Autodesk Inventor part; units mm, degrees
ref_plane "YZ Plane" through (0, 0, 0) normal (1, 0, 0) x (0, 1, 0)
ref_plane "XZ Plane" through (0, 0, 0) normal (0, 1, 0) x (-1, 0, 0)
ref_plane "XY Plane" through (0, 0, 0) normal (0, 0, 1) x (1, 0, 0)
sketch "Boceto1" plane through (0, 0, 0) normal (0, 0, 1) x (1, 0, 0)
  line L0 (30, -83.65) -> (30, 0)
  line L1 (0, 0) -> (30, 0)
  line L2 (0, 0) -> (0, -83.65)
  line L3 (0, -83.65) -> (30, -83.65)
  line L4 (-13.92, -24.65) -> (-9.92, -24.65)
  line L5 (30, -83.65) -> (-55, -83.65)
  line L6 (-55, -83.65) -> (-55, -24.65)
  line L7 (-55, -24.65) -> (30, -24.65)
  line L8 (30, -24.65) -> (30, -83.65)
  line L9 (-55, -24.65) -> (-55, -21.65)
  line L10 (-55, -21.65) -> (30, -21.65)
  line L11 (0, -83.65) -> (10, -83.65)
  line L12 (10, -83.65) -> (10, -21.65)
  circle A0 centre (5, -78.65) radius 2.1
  circle A1 centre (5, -26.65) radius 2.1
  dimension "d0" = 85
  dimension "d1" = 59
  dimension "d2" = 3
  dimension "d5" = 10
extrude "Extrusión1" add sketch "Boceto1" along normal blind 6 contours L3 L2 L7 A1 L12 | L7 A1 L2 L10 L12 | L5 L6 L7 L4 L2 | A1 L7 | L7 A1 | L7 L4 L9 L10 L2 | A0
sketch "Boceto2" plane through (0, 0, 6) normal (0, 0, 1) x (1, 0, 0)
  line L0 (10, -83.65) -> (10, -21.65)
  line L1 (-55, -83.65) -> (10, -83.65)
  line L2 (10, -21.65) -> (-55, -21.65)
  point P0 (0, 0)
  point P1 (5, -78.65)
  point P2 (5, -26.65)
  dimension "d6" = 5
  dimension "d7" = 5
  dimension "d8" = 5
  dimension "d9" = 5
hole "Agujero1" at (5, -78.65, 6) at (5, -26.65, 6) direction (0, 0, -1) diameter 3.2 end through all
sketch "Boceto3" plane through (0, 0, 0) normal (0, 0, -1) x (-1, 0, 0)
  circle A0 centre (-5, -78.65) radius 2.1
  circle A1 centre (-5, -26.65) radius 2.1
  line L0 (-12, 0) -> (-12, -7.15)
  line L1 (-12, -7.15) -> (-30, -7.15)
  line L2 (-30, -7.15) -> (-30, -83.65)
  line L3 (0, -83.65) -> (-30, -83.65)
  line L4 (0, -83.65) -> (0, 0)
  line L5 (0, 0) -> (-12, 0)
  line L6 (20.12, -21.65) -> (-10, -21.65)
  line L7 (-10, -21.65) -> (-10, -83.65)
  circle A2 centre (-5, -26.65) radius 1.6
  circle A3 centre (-5, -78.65) radius 1.6
  circle A4 centre (-5, -26.65) radius 1.6
  circle A5 centre (-5, -78.65) radius 1.6
  line L8 (55, -21.65) -> (55, -83.65)
  line L9 (-10, -21.65) -> (55, -21.65)
  line L10 (-10, -83.65) -> (-10, -21.65)
  line L11 (55, -83.65) -> (-10, -83.65)
  line L12 (-10, -83.65) -> (20.12, -83.65)
  line L13 (20.12, -83.65) -> (20.12, -21.65)
  point P0 (0, -21.65)
extrude "Extrusión2" cut sketch "Boceto3" against normal blind 3 contours A0 | A1 | L5 L4 L6 L7 L3 L2 L1 L0 | L6 L13 L11 L4 | L4 L3 L7 L6 | L9 L8 L11 L13 | A2 | A3
sketch "Boceto4" plane through (-55, -21.65, 6) normal (0, 1, 0) x (1, 0, 0)
  line L0 (65, 3) -> (0, 3)
  line L1 (0, 3) -> (0, 0)
  line L2 (65, 0) -> (0, 0)
  line L3 (65, 3) -> (65, 0)
  line L4 (0, 0) -> (65, 0)
  line L5 (65, 0) -> (65, 6)
  line L6 (65, 6) -> (0, 6)
  line L7 (0, 6) -> (0, 0)
  point P0 (55, 6)
extrude "Extrusión3" add sketch "Boceto4" along normal blind 5
sketch "Boceto5" plane through (-55, -83.65, 3) normal (-1, 0, 0) x (0, 0, 1)
  line L0 (-69, 62) -> (-69, 59)
  line L1 (-3, 59) -> (-69, 59)
  line L2 (-3, 59) -> (-3, 62)
  line L3 (-3, 62) -> (-69, 62)
  line L4 (0, 62) -> (0, 0)
  line L5 (0, 0) -> (3, 0)
  line L6 (3, 0) -> (3, 67)
  line L7 (-3, 67) -> (3, 67)
  line L8 (-3, 62) -> (-3, 67)
  line L9 (-3, 62) -> (0, 62)
  line L10 (-3, 59) -> (3, 59)
  line L11 (3, 59) -> (3, 62)
  line L12 (3, 62) -> (-3, 62)
  line L13 (-3, 62) -> (-3, 59)
  point P0 (-3, 83.65)
  point P1 (0, 59)
extrude "Extrusión4" cut sketch "Boceto5" against normal blind 33.88 contours L12 L6 L10 L4
sketch "Boceto6" plane through (-55, -16.65, 6) normal (0, 1, 0) x (1, 0, 0)
  line L0 (0, 6) -> (0, 0)
  line L1 (0, 0) -> (65, 0)
  line L2 (65, 0) -> (65, 6)
  line L3 (65, 6) -> (0, 6)
  line L4 (0, 0) -> (0, 3)
  line L5 (0, 3) -> (3, 3)
  circle A0 centre (3, 3) radius 2.1
  line L6 (33.88, 3) -> (33.88, 0)
  line L7 (33.88, 3) -> (30.88, 3)
  circle A1 centre (30.88, 3) radius 2.1
  dimension "d34" = 3
  dimension "d35" = 4.2
  dimension "d36" = 4.2
hole "Agujero2" at (-52, -16.65, 3) at (-24.12, -16.65, 3) direction (0, -1, 0) diameter 4.2 depth 5
properties part number "Lateral izquierdo"
Input: part model. Units: mm. Frame: model coordinates. A direction names the side the tool comes from. Coordinates: 2 decimals unless noted, no trailing zeros. Write each loop counter-clockwise with the first axis right and the second up, starting at its lowest first coordinate (ties: lowest second). Pieces come first, ordered by that corner, then holes. Notation, with made-up numbers: M 84,-6 L 135,-6 A15 ccw 135,16 Z; hole C 79,28 d10. An arc over 180 degrees is marked long. Answer as a JSON object with one key per item and string values. Group by question number.
(1) Section A-A on x = 5. Output: boundary loops of the cut face in (y, z), plus the area to 3 significant figures.
(2) Section C-C on x = -40. Output: boundary loops of the cut face in (y, z).
(3) Mould query, pull axis Y, two halves, no side actions, for faces 4 (the face through (4.93, -77.05, 4.48)), 5 (the face through (-22.257, -19.185, 3.969)), 6 (the face through (-23, -16.65, 1)). Classes: pulls with the +Y half, pulls with the -Y half, needs draft (parallel to the pull), parting line crosses it, or undercut.
(4) Ray query, line 1 along X through (y, z) = (-18.1, 3); line 2 along Y through (x, z) = (5, 3.75); line 3 along X through (y, z) = (-26.65, 4). Return the intervals inside material, ascending. Write a range as [from, to].
(5) Section B-B on y = -26.65. Output: boundary loops of the cut face in (x, z).
(6) Section D-D on x = -24.12. Output: boundary loops of the cut face in (y, z).
(7) Set-up query: faces 1 (the face through (-22, -52, 3)), 2 (the face through (-23, -21.65, 1)), 3 (the face through (-21.12, -23, 4)). Return all of +Z, -Z, +X, -X, +Y, -Y with unobstructed straight access to the full face (end or side cutting, diameter ignored); none if empty.
(8) Contact query for flat-ended pins moving along their axis: P1, Ø4, axis at x = 5, y = -78.65, coming from the -Z side; P2, Ø2.5, axis at y = -23, z = 4, coming from the -X side. Output: stop coordinate, or through.
Result set:
{
 "1": {"outline": "M -83.65,3 L -80.25,3 L -80.25,6 L -83.65,6 Z; M -77.05,3 L -28.25,3 L -28.25,6 L -77.05,6 Z; M -25.05,3 L -21.65,3 L -21.65,0 L -16.65,0 L -16.65,6 L -25.05,6 Z", "area": "197 mm2"},
 "2": {"outline": "M -83.65,3 L -24.65,3 L -24.65,6 L -83.65,6 Z; M -21.65,0 L -16.65,0 L -16.65,6 L -21.65,6 Z"},
 "3": {"face 4": "undercut", "face 5": "needs draft", "face 6": "pulls with the +Y half"},
 "4": {"line 1": "x = [-55, -54.1], [-49.9, -26.22], [-22.02, 10]", "line 2": "y = [-83.65, -80.25], [-77.05, -28.25], [-25.05, -16.65]", "line 3": "x = [-55, 3.4], [6.6, 10]"},
 "5": {"outline": "M -55,3 L 3.4,3 L 3.4,6 L -55,6 Z; M 6.6,3 L 10,3 L 10,6 L 6.6,6 Z"},
 "6": {"outline": "M -83.65,3 L -24.65,3 L -24.65,6 L -83.65,6 Z; M -21.65,0 L -16.65,0 L -16.65,0.9 L -21.65,0.9 Z; M -21.65,5.1 L -16.65,5.1 L -16.65,6 L -21.65,6 Z"},
 "7": {"face 1": "-Z, +X, -X, -Y", "face 2": "-Z, -X", "face 3": "+Z, -Z, -X"},
 "8": {"P1": "stops at z = 3", "P2": "stops at x = -21.12"}
}
